Can you work these out from the model? Positions are in its coordinate system, mm. A direction names the side the tool comes from. Give positions to 0.01 mm unless a question says otherwise; leave off trailing zeros. Loops run counter-clockwise (first coordinate to the right, second up) from the corner with the lowest first, then second, coordinate; pieces in that order, holes last. Notation, with made-up numbers: M -29,51.25 L 2,51.25 A28 ccw 2,75.25 Z; hole C 5,19 d2. An arc over 180 degrees is marked long. One line per item, written item: value. Start each with the question number.
from build123d import *

# Parameters (mm, degrees)
BOSS_EXTRUDE1_DEPTH = 1.5875
FILLET1_R           = 3.175


with BuildPart() as part:
    # Sketch4 → Boss-Extrude1 (new body)
    with BuildSketch(Plane.XY):
        with BuildLine():
            Line((100.453077844, 80.395193317), (94.322399388, 79.923602666))
            ThreePointArc((94.322399388, 79.923602666), (80.150110348, 79.621122729), (88.821616455, 68.40728072))
            Line((88.821616455, 68.40728072), (87.008390154, 74.451368388))
            Line((87.008390154, 74.451368388), (87.768664768, 74.679450772))
            Line((87.768664768, 74.679450772), (88.528939382, 74.907533156))
            Line((88.528939382, 74.907533156), (90.342165683, 68.863445488))
            ThreePointArc((90.342165683, 68.863445488), (93.082490895, 70.749210028), (94.809422156, 73.592306683))
            Line((94.809422156, 73.592306683), (100.940100612, 74.063897334))
            ThreePointArc((100.940100612, 74.063897334), (104.003334801, 70.900719906), (108.281132842, 69.856910029))
            Line((108.281132842, 69.856910029), (107.388733992, 76.103701977))
            Line((107.388733992, 76.103701977), (108.174506403, 76.215955179))
            Line((108.174506403, 76.215955179), (108.960278814, 76.32820838))
            Line((108.960278814, 76.32820838), (109.852677663, 70.081416432))
            ThreePointArc((109.852677663, 70.081416432), (112.484101458, 71.272453552), (114.515120736, 73.3262114))
            Line((114.515120736, 73.3262114), (125.614647067, 71.245050213))
            ThreePointArc((125.614647067, 71.245050213), (128.101842683, 67.070106968), (132.55625, 65.127287218))
            Line((132.55625, 65.127287218), (132.55625, 71.477287218))
            Line((132.55625, 71.477287218), (133.35, 71.477287218))
            Line((133.35, 71.477287218), (134.14375, 71.477287218))
            Line((134.14375, 71.477287218), (134.14375, 65.127287218))
            ThreePointArc((134.14375, 65.127287218), (136.675698551, 65.817806691), (138.844082076, 67.296215802))
            Line((138.844082076, 67.296215802), (144.463610232, 64.954745737))
            ThreePointArc((144.463610232, 64.954745737), (146.356207306, 59.941970278), (151.002861083, 57.273927891))
            Line((151.002861083, 57.273927891), (151.48988385, 63.605223874))
            Line((151.48988385, 63.605223874), (152.281295848, 63.544346028))
            Line((152.281295848, 63.544346028), (153.072707846, 63.483468182))
            Line((153.072707846, 63.483468182), (152.585685078, 57.152172199))
            ThreePointArc((152.585685078, 57.152172199), (159.729512866, 68.134161681), (146.905917924, 70.816284198))
            Line((146.905917924, 70.816284198), (141.286389768, 73.157754263))
            ThreePointArc((141.286389768, 73.157754263), (135.620274668, 80.630902917), (126.784879264, 77.4862886))
            Line((126.784879264, 77.4862886), (115.685352934, 79.567449787))
            ThreePointArc((115.685352934, 79.567449787), (108.380699601, 85.713306212), (100.453077844, 80.395193317))
        make_face()
        with BuildLine():
            ThreePointArc((134.354023157, 76.037069471), (133.228154551, 76.197661136), (132.117919025, 75.951192316))
            Line((132.117919025, 75.951192316), (130.654822867, 75.335151828))
            Line((130.654822867, 75.335151828), (129.422741892, 78.261344145))
            Line((129.422741892, 78.261344145), (130.88583805, 78.877384632))
            ThreePointArc((130.88583805, 78.877384632), (133.106309101, 79.370322273), (135.358046314, 79.049138943))
            Line((135.358046314, 79.049138943), (136.86408105, 78.547127364))
            Line((136.86408105, 78.547127364), (135.860057893, 75.535057893))
            Line((135.860057893, 75.535057893), (134.354023157, 76.037069471))
        make_face(mode=Mode.SUBTRACT)
        with BuildLine():
            ThreePointArc((83.557340736, 81.320671724), (86.234149214, 82.457767939), (89.137159073, 82.282196911))
            Line((89.137159073, 82.282196911), (90.657708301, 81.826032143))
            Line((90.657708301, 81.826032143), (89.745378764, 78.784933687))
            Line((89.745378764, 78.784933687), (88.224829537, 79.241098456))
            ThreePointArc((88.224829537, 79.241098456), (86.773324607, 79.32888397), (85.434920368, 78.760335862))
            Line((85.434920368, 78.760335862), (84.154752437, 77.821546046))
            Line((84.154752437, 77.821546046), (82.277172805, 80.381881908))
            Line((82.277172805, 80.381881908), (83.557340736, 81.320671724))
        make_face(mode=Mode.SUBTRACT)
        with BuildLine():
            ThreePointArc((109.182080975, 80.713692316), (107.712055506, 80.953571291), (106.29439622, 80.496669822))
            Line((106.29439622, 80.496669822), (104.939811309, 79.668867932))
            Line((104.939811309, 79.668867932), (103.284207529, 82.378037754))
            Line((103.284207529, 82.378037754), (104.63879244, 83.205839644))
            ThreePointArc((104.63879244, 83.205839644), (107.474111012, 84.119642581), (110.41416195, 83.639884632))
            Line((110.41416195, 83.639884632), (111.877258108, 83.023844145))
            Line((111.877258108, 83.023844145), (110.645177133, 80.097651828))
            Line((110.645177133, 80.097651828), (109.182080975, 80.713692316))
        make_face(mode=Mode.SUBTRACT)
        with BuildLine():
            ThreePointArc((154.612294548, 67.364862034), (153.086943568, 68.187295725), (151.356947016, 68.08627733))
            Line((151.356947016, 68.08627733), (149.857558351, 67.564750837))
            Line((149.857558351, 67.564750837), (148.814505367, 70.563528167))
            Line((148.814505367, 70.563528167), (150.313894032, 71.085054659))
            ThreePointArc((150.313894032, 71.085054659), (153.773887136, 71.287091449), (156.824589095, 69.642224068))
            Line((156.824589095, 69.642224068), (157.963270112, 68.536076795))
            Line((157.963270112, 68.536076795), (155.750975565, 66.25871476))
            Line((155.750975565, 66.25871476), (154.612294548, 67.364862034))
        make_face(mode=Mode.SUBTRACT)
    extrude(amount=BOSS_EXTRUDE1_DEPTH)

    # Fillet1
    fillet1_edges = [part.edges().sort_by_distance(p)[0] for p in [
        (94.322399388, 79.923602666, 0.79375),
        (100.453077844, 80.395193317, 0.79375),
        (115.685352934, 79.567449787, 0.79375),
        (126.784879264, 77.4862886, 0.79375),
        (141.286389768, 73.157754263, 0.79375),
        (146.905917924, 70.816284198, 0.79375),
        (144.463610232, 64.954745737, 0.79375),
        (138.844082076, 67.296215802, 0.79375),
        (125.614647067, 71.245050213, 0.79375),
        (114.515120736, 73.3262114, 0.79375),
        (100.940100612, 74.063897334, 0.79375),
        (94.809422156, 73.592306683, 0.79375),
    ]]
    fillet(fillet1_edges, radius=FILLET1_R)


solid = part.part
Q1. I need wall thicknesses on line 1 along X through (y, z) = (81.25, 0.5); line 2 along X through (y, z) = (82.75, 1.45); line 3 along X through (y, z) = (79.5, 0.1). Which ranges of each line are inside material? Lowest first, please.
Q2. If we mould it in two halves opening along Y, with no side actions, what happens to faces 4 (the face through (132.556, 68, 1)), 5 (the face through (139.07, 66.82, 0.8)), 6 (the face through (87.758, 74.676, 0.783))? For each: released by +Y, released by -Y, zero draft, split by the parting line, or undercut.
Q3. For P1, Ø4, axis at x = 88, y = 81, coming from the +Z side; P2, Ø10, axis at x = 148, y = 79.5, coming from the +Z side, each with a flat end and sliding along its axis, tell me the tip position at first contact or that it passes through.
Q4. If we section it at A-A, the plane y = 61.25: Write out the boundary of the cut face in (x, z), plus the area to 3 significant figures.
Q5. If we section it at B-B, the plane z = 0.8: Give the number of separate pieces and of enclosed holes in the cut face, plus the area to 3 significant figures.
Q6. Which directions (+Z, -Z, +X, -X, +Y, -Y) give clear straight access to the entire face, cutting with the end or side of a thin tool? Please do faces 1 (the face through (121.287, 78.517, 0.783)), 2 (the face through (125.163, 70.973, 0.805)), 3 (the face through (83.23, 79.08, 0.78)).
Response:
1. line 1: 81.19 to 83.46, 90.48 to 93.44, 100.69 to 103.97, 111.13 to 115.09
1. line 2: 82.83 to 91.8, 101.76 to 103.89, 111.76 to 114.14
1. line 3: 80.09 to 82.92, 89.96 to 116.68, 128.76 to 137.94
2. face 4: zero draft
2. face 5: released by -Y
2. face 6: undercut
3. P1: z = 1.59
3. P2: through
4. outline: M 145.45,0 L 151.31,0 L 151.31,1.59 L 145.45,1.59 Z; M 152.9,0 L 159.35,0 L 159.35,1.59 L 152.9,1.59 Z
4. area: 19.5 mm^2
5. separate pieces: 1
5. enclosed holes: 4
5. area: 794 mm^2
6. face 1: +Z, -Z, +Y
6. face 2: +Z, -Z, -Y
6. face 3: +Z, -Z
